The figure shows three views and two pictorial views of one solid part (mm, origin at its lowest corner). Answer the questions. Coordinates: 2 decimals unless noted, no trailing zeros. Order: outer loops, then holes, each group sorted by start corner. A loop starts at its lowest first (then second) coordinate and runs counter-clockwise, first axis right, second up. Notation, with made-up numbers: (8, 43) -> (63, 43) arc R12 cw to (63, 60) -> close; hole circle Ø9 at (-27.5, -19.5). An arc over 180 degrees is marked (long way). Return JSON: item names as keys, results as strings. Group by question number.
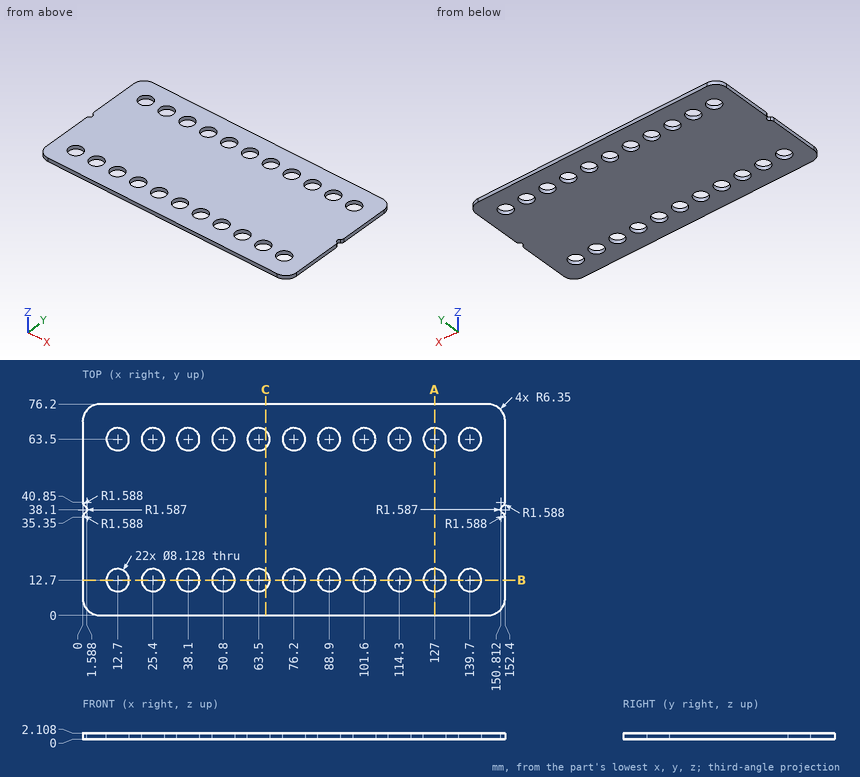
1. Find section A-A on x = 127. Determine the outline of the cut face in (y, z) (1 decimal).
2. Find section C-C on x = 66. Determine the outline of the cut face in (y, z) (1 decimal).
3. Straight lines are drawn through the part: L1, parallel to Y at x = 139.7, z = 0.6 (1 decimal); L2, parallel to Y at x = 47.5, z = 0.9 (1 decimal); L3, parallel to X at y = 40, z = 1.15 (1 decimal). For each, find the intervals that lie inside material, in ascending order.
4. Find section B-B on y = 12.7. Give the number of separate pieces and of enclosed holes in the cut face, and give its area (3 significant figures).
Result:
{
 "1": {"outline": "(0, 0) -> (8.6, 0) -> (8.6, 2.1) -> (0, 2.1) -> close; (16.8, 0) -> (59.4, 0) -> (59.4, 2.1) -> (16.8, 2.1) -> close; (67.6, 0) -> (76.2, 0) -> (76.2, 2.1) -> (67.6, 2.1) -> close"},
 "2": {"outline": "(0, 0) -> (9.5, 0) -> (9.5, 2.1) -> (0, 2.1) -> close; (15.9, 0) -> (60.3, 0) -> (60.3, 2.1) -> (15.9, 2.1) -> close; (66.7, 0) -> (76.2, 0) -> (76.2, 2.1) -> (66.7, 2.1) -> close"},
 "3": {"L1": "0 to 8.6, 16.8 to 59.4, 67.6 to 76.2", "L2": "0 to 10.3, 15.1 to 61.1, 65.9 to 76.2", "L3": "0.2 to 152.2"},
 "4": {"separate pieces": "12", "enclosed holes": "0", "area": "133 mm^2"}
}
